Answer from the drawing. Dimensions are ordinates in mm from the lowest x, y and z of the part. Round coordinates to 2 decimals unless told otherwise and drop trailing zeros. Loops run counter-clockwise (first coordinate to the right, second up) from the corner with the lowest first, then second, coordinate; pieces in that order, holes last. Notation, with made-up numbers: (60, 2.5) -> (83, 2.5) arc R15 ccw to (83, 25.5) -> close; hole circle Ø10 at (72.5, 51). An arc over 180 degrees is marked (long way). Use CSV: the item, a comma, the result in double quotes. Start each with the question number.
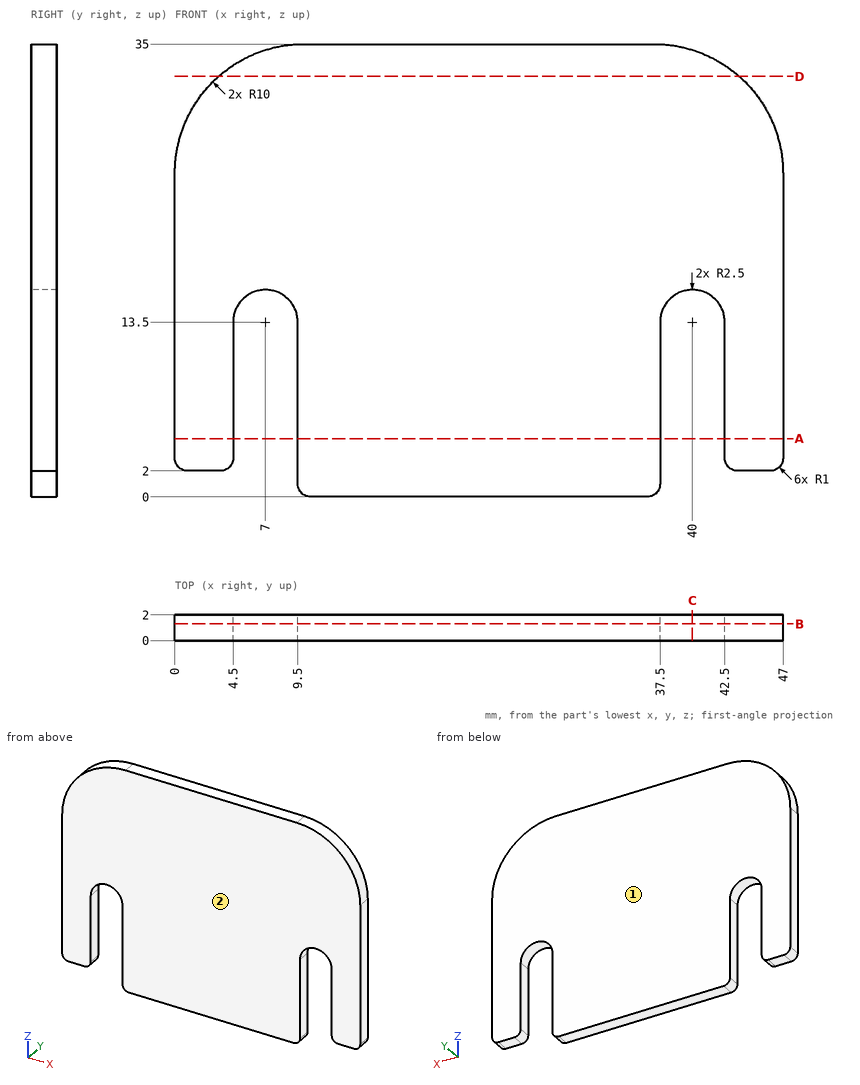
Q1. Section B-B, the plane y = 1.3 is taken. Write down the section's boundary in (x, z).
Q2. This flat-tipped pin is pushed along its axis until it touches: pin 1 (1 mm diameter, centred on x = 45, y = 1, fed in from -Z). Where does it stop, or does it pass through?
Q3. Straight lines are drawn through the part: line 1 (X direction, y = 1.7, z = 8.5); line 2 (Z direction, x = 6.5, y = 1.8); line 3 (X direction, y = 1.45, z = 29.5). For each, find the intervals that lie inside material, in ascending order. Write a range as from..to.
Q4. Section C-C, the plane x = 40 is taken. Write down the section's boundary in (y, z).
Q5. Section D-D, the plane z = 32.5 is taken. Write down the section's boundary in (x, y), and give its area (3 significant figures).
Q6. For a pull along Y with two mould halves and no side action, classify the marked faces 1 and 2 as pulls with the +Y half, pulls with the -Y half, needs draft (parallel to the pull), parting line crosses it, or undercut.
Q7. Section A-A, the plane z = 4.5 is taken. Write down the section's boundary in (x, y).
Report:
1,outline,"(0, 3) arc R1 ccw to (1, 2) -> (3.5, 2) arc R1 ccw to (4.5, 3) -> (4.5, 13.5) arc R2.5 cw to (9.5, 13.5) -> (9.5, 1) arc R1 ccw to (10.5, 0) -> (36.5, 0) arc R1 ccw to (37.5, 1) -> (37.5, 13.5) arc R2.5 cw to (42.5, 13.5) -> (42.5, 3) arc R1 ccw to (43.5, 2) -> (46, 2) arc R1 ccw to (47, 3) -> (47, 25) arc R10 ccw to (37, 35) -> (10, 35) arc R10 ccw to (0, 25) -> close"
2,pin 1,"stops at z = 2"
3,line 1,"x = 0..4.5, 9.5..37.5, 42.5..47"
3,line 2,"z = 15.95..34.37"
3,line 3,"x = 1.07..45.93"
4,outline,"(0, 16) -> (2, 16) -> (2, 34.54) -> (0, 34.54) -> close"
5,outline,"(3.39, 0) -> (43.61, 0) -> (43.61, 2) -> (3.39, 2) -> close"
5,area,"80.5 mm²"
6,face 1,"pulls with the +Y half"
6,face 2,"pulls with the -Y half"
7,outline,"(0, 0) -> (4.5, 0) -> (4.5, 2) -> (0, 2) -> close; (9.5, 0) -> (37.5, 0) -> (37.5, 2) -> (9.5, 2) -> close; (42.5, 0) -> (47, 0) -> (47, 2) -> (42.5, 2) -> close"
